Verification items for the finished model (mm, model axes). A direction names the side the tool comes from. Coordinates: 2 decimals unless noted, no trailing zeros. Order: outer loops, then holes, each group sorted by start corner. A loop starts at its lowest first (then second) coordinate and runs counter-clockwise, first axis right, second up. Notation, with made-up numbers: M 81.5,67 L 113.5,67 A14 cw 113.5,88 Z; hole C -12.75,14 d2. An arc over 180 degrees is marked long. Return JSON: item names as keys, results as strings. Group by question number.
1. Material ranges on line 1 along Y through (x, z) = (16, 1.55); line 2 along X through (y, z) = (-18, 3.2); line 3 along Y through (x, z) = (-15.5, 4.2), recorded low to high.
2. Gauge pin test, flat ends, axial feed: pin 1 (1.1 mm diameter, centred on x = 23, z = 2, fed in from -Y); pin 2 (3.5 mm diameter, centred on x = -16.02, y = 16.02, fed in from +Z); pin 3 (3 mm diameter, centred on y = -22.5, z = 2, fed in from +X). Record the tip position at first contact, or that the pin passes through.
3. Mould release check, pull along X, two halves, no side actions. Record for faces 1 (the cylindrical face through (-13.336, 16.616, 3.479)), 2 (the flat face through (-5.9, 11.4, 5)), 3 (the flat face through (-24.901, 0, 2)): +X half, -X half, draft (parallel to the pull), parting line (faces both ways), or undercut.
4. Section check C-C, the plane z = 1.15. Record the cut outline in (x, y), plus the area to 3 significant figures.
5. Section check B-B, the plane y = 0. Record the cut outline in (x, z).
6. Section check D-D, the plane x = 20. Record the cut outline in (y, z).
7. Section check A-A, the plane x = 7.5. Record the cut outline in (y, z), plus the area to 3 significant figures.
8. Set-up check for faces 4 (the cylindrical face through (-13.58, -17.29, 3.48)), 5 (the flat face through (24.901, 0, 2)), 6 (the flat face through (-17, -23, 3)), 7 (the flat face through (23, 17, 3)): record each of +Z, -Z, +X, -X, +Y, -Y from which the full face is reachable in a straight line by a thin tool's end or side.
Autodesk Inventor part; units mm, degrees
ref_plane "YZ Plane" through (0, 0, 0) normal (1, 0, 0) x (0, 1, 0)
ref_plane "XZ Plane" through (0, 0, 0) normal (0, 1, 0) x (-1, 0, 0)
ref_plane "XY Plane" through (0, 0, 0) normal (0, 0, 1) x (1, 0, 0)
sketch "Sketch1" plane through (0, 0, 0) normal (0, 0, 1) x (1, 0, 0)
  line L0 (-39.3843, 0) -> (62.0012, 0) construction
  line L1 (0, -36.6008) -> (0, 45.3001) construction
  line L2 (0, 0) -> (33.6, 33.6) construction
  line L3 (0, 0) -> (47.5176, 0) construction
  line L4 (0, 24.9006) -> (16.8, 24.9006)
  line L5 (16.8, 24.9006) -> (16.8, 21.2406)
  line L6 (16.8, 21.2406) -> (19.0203, 19.0203)
  line L7 (24.9006, 0) -> (24.9006, 16.8)
  line L8 (24.9006, 16.8) -> (21.2406, 16.8)
  line L9 (21.2406, 16.8) -> (19.0203, 19.0203)
  line L10 (0, 24.9006) -> (-16.8, 24.9006)
  line L11 (-16.8, 24.9006) -> (-16.8, 21.2406)
  line L12 (-16.8, 21.2406) -> (-19.0203, 19.0203)
  line L13 (-24.9006, 0) -> (-24.9006, 16.8)
  line L14 (-24.9006, 16.8) -> (-21.2406, 16.8)
  line L15 (-21.2406, 16.8) -> (-19.0203, 19.0203)
  line L16 (0, -24.9006) -> (16.8, -24.9006)
  line L17 (16.8, -24.9006) -> (16.8, -21.2406)
  line L18 (16.8, -21.2406) -> (19.0203, -19.0203)
  line L19 (24.9006, 0) -> (24.9006, -16.8)
  line L20 (24.9006, -16.8) -> (21.2406, -16.8)
  line L21 (21.2406, -16.8) -> (19.0203, -19.0203)
  line L22 (0, -24.9006) -> (-16.8, -24.9006)
  line L23 (-16.8, -24.9006) -> (-16.8, -21.2406)
  line L24 (-16.8, -21.2406) -> (-19.0203, -19.0203)
  line L25 (-24.9006, 0) -> (-24.9006, -16.8)
  line L26 (-24.9006, -16.8) -> (-21.2406, -16.8)
  line L27 (-21.2406, -16.8) -> (-19.0203, -19.0203)
  circle A0 centre (0, 0) radius 12.5
  dimension "d0" = 45
  dimension "d1" = 16.8
  dimension "d2" = 3.66
  dimension "d3" = 3.14
  dimension "d4" = 25
extrude "Extrusion1" add sketch "Sketch1" along normal blind 5
sketch "Sketch2" plane through (0, 0, 5) normal (0, 0, 1) x (1, 0, 0)
  circle A0 centre (0, 0) radius 12.5 construction
  line L0 (16.8, 24.9006) -> (-16.8, 24.9006) construction
  line L1 (-16.8, 24.9006) -> (-16.8, 21.2406) construction
  line L2 (-16.8, 21.2406) -> (-21.2406, 16.8) construction
  line L3 (-21.2406, 16.8) -> (-24.9006, 16.8) construction
  line L4 (-24.9006, 16.8) -> (-24.9006, -16.8) construction
  line L5 (-24.9006, -16.8) -> (-21.2406, -16.8) construction
  line L6 (-21.2406, -16.8) -> (-16.8, -21.2406) construction
  line L7 (-16.8, -21.2406) -> (-16.8, -24.9006) construction
  line L8 (-16.8, -24.9006) -> (16.8, -24.9006) construction
  line L9 (16.8, -24.9006) -> (16.8, -21.2406) construction
  line L10 (16.8, -21.2406) -> (21.2406, -16.8) construction
  line L11 (21.2406, -16.8) -> (24.9006, -16.8) construction
  line L12 (24.9006, -16.8) -> (24.9006, 16.8) construction
  line L13 (24.9006, 16.8) -> (21.2406, 16.8) construction
  line L14 (21.2406, 16.8) -> (16.8, 21.2406) construction
  line L15 (16.8, 21.2406) -> (16.8, 24.9006) construction
  circle A1 centre (16.0203, -16.0203) radius 2.1846 construction
  circle A2 centre (-16.0203, -16.0203) radius 2.1846 construction
  circle A3 centre (-16.0203, 16.0203) radius 2.1846 construction
  circle A4 centre (16.0203, 16.0203) radius 2.1846 construction
  circle A5 centre (0, 0) radius 14 construction
  line L16 (-19.0203, 17.0203) -> (-19.0203, -17.0203) construction
  arc A6 (-17.0203, 19.0203) -> (-19.0203, 17.0203) centre (-17.0203, 17.0203) ccw construction
  line L17 (17.0203, 19.0203) -> (-17.0203, 19.0203) construction
  arc A7 (19.0203, 17.0203) -> (17.0203, 19.0203) centre (17.0203, 17.0203) ccw construction
  line L18 (19.0203, -17.0203) -> (19.0203, 17.0203) construction
  arc A8 (17.0203, -19.0203) -> (19.0203, -17.0203) centre (17.0203, -17.0203) ccw construction
  line L19 (-17.0203, -19.0203) -> (17.0203, -19.0203) construction
  arc A9 (-19.0203, -17.0203) -> (-17.0203, -19.0203) centre (-17.0203, -17.0203) ccw construction
hole "Hole1" at (-16.0203, 16.0203, 5) at (16.0203, 16.0203, 5) at (16.0203, -16.0203, 5) at (-16.0203, -16.0203, 5) direction (0, 0, -1) diameter 2.8 end through all counterbore diameter 5.5 counterbore depth 3
sketch "Skizze3" plane through (0, 0, 5) normal (0, 0, 1) x (1, 0, 0)
  circle A0 centre (16.0203, -16.0203) radius 2.75 construction
  circle A1 centre (-16.0203, 16.0203) radius 2.75 construction
  circle A2 centre (16.0203, 16.0203) radius 2.75 construction
  circle A3 centre (-16.0203, -16.0203) radius 2.75 construction
  circle A4 centre (0, 0) radius 12.5 construction
  line L0 (16.8, 24.9006) -> (-16.8, 24.9006) construction
  line L1 (-16.8, 24.9006) -> (-16.8, 21.2406)
  line L2 (-16.8, 21.2406) -> (-21.2406, 16.8)
  line L3 (-21.2406, 16.8) -> (-24.9006, 16.8)
  line L4 (-24.9006, 16.8) -> (-24.9006, -16.8) construction
  line L5 (-24.9006, -16.8) -> (-21.2406, -16.8)
  line L6 (-21.2406, -16.8) -> (-16.8, -21.2406)
  line L7 (-16.8, -21.2406) -> (-16.8, -24.9006)
  line L8 (-16.8, -24.9006) -> (16.8, -24.9006) construction
  line L9 (16.8, -24.9006) -> (16.8, -21.2406)
  line L10 (16.8, -21.2406) -> (21.2406, -16.8)
  line L11 (21.2406, -16.8) -> (24.9006, -16.8)
  line L12 (24.9006, -16.8) -> (24.9006, 16.8) construction
  line L13 (24.9006, 16.8) -> (21.2406, 16.8)
  line L14 (21.2406, 16.8) -> (16.8, 21.2406)
  line L15 (16.8, 21.2406) -> (16.8, 24.9006)
  line L16 (-17, 25.1006) -> (17, 25.1006) construction
  line L17 (17, 25.1006) -> (17, 21.3235)
  line L18 (17, 21.3235) -> (21.3235, 17)
  line L19 (21.3235, 17) -> (25.1006, 17)
  line L20 (25.1006, 17) -> (25.1006, -17) construction
  line L21 (25.1006, -17) -> (21.3235, -17)
  line L22 (21.3235, -17) -> (17, -21.3235)
  line L23 (17, -21.3235) -> (17, -25.1006)
  line L24 (17, -25.1006) -> (-17, -25.1006) construction
  line L25 (-17, -25.1006) -> (-17, -21.3235)
  line L26 (-17, -21.3235) -> (-21.3235, -17)
  line L27 (-21.3235, -17) -> (-25.1006, -17)
  line L28 (-25.1006, -17) -> (-25.1006, 17) construction
  line L29 (-25.1006, 17) -> (-21.3235, 17)
  line L30 (-21.3235, 17) -> (-17, 21.3235)
  line L31 (-17, 21.3235) -> (-17, 25.1006)
  line L32 (-24.9006, 16.8) -> (-24.9006, 17)
  line L33 (-16.8, 24.9006) -> (-17, 24.9006)
  line L34 (16.8, 24.9006) -> (17, 24.9006)
  line L35 (24.9006, 16.8) -> (24.9006, 17)
  line L36 (24.9006, -16.8) -> (24.9006, -17)
  line L37 (16.8, -24.9006) -> (16.8, -21.2406)
  line L38 (16.8, -24.9006) -> (17, -24.9006)
  line L39 (-16.8, -24.9006) -> (-17, -24.9006)
  line L40 (-24.9006, -16.8) -> (-24.9006, -17)
  dimension "d14" = 0.2
extrude "IM_offset" add sketch "Skizze3" against normal up to surface (5 mm away)
properties part number "20_Cube_insert_Sample_holder_magnetic_v3"
Answers follow:
{
 "1": {"line 1": "-24.9 to -17.42, -14.62 to 14.62, 17.42 to 24.9", "line 2": "-20.32 to -17.93, -14.11 to 14.11, 17.93 to 20.32", "line 3": "-24.9 to -18.72, -13.32 to 13.32, 18.72 to 24.9"},
 "2": {"pin 1": "y = -17", "pin 2": "z = 2", "pin 3": "x = 17.32"},
 "3": {"face 1": "undercut", "face 2": "draft", "face 3": "-X half"},
 "4": {"outline": "M -24.9,-17 L -21.32,-17 L -17,-21.32 L -17,-24.9 L 17,-24.9 L 17,-21.32 L 21.32,-17 L 24.9,-17 L 24.9,17 L 21.32,17 L 17,21.32 L 17,24.9 L -17,24.9 L -17,21.32 L -21.32,17 L -24.9,17 Z; hole C -16.02,-16.02 d2.8; hole C -16.02,16.02 d2.8; hole C 0,0 d25; hole C 16.02,-16.02 d2.8; hole C 16.02,16.02 d2.8", "area": "1,750 mm^2"},
 "5": {"outline": "M -24.9,0 L -12.5,0 L -12.5,5 L -24.9,5 Z; M 12.5,0 L 24.9,0 L 24.9,5 L 12.5,5 Z"},
 "6": {"outline": "M -18.32,0 L 18.32,0 L 18.32,5 L -18.32,5 Z"},
 "7": {"outline": "M -24.9,0 L -10,0 L -10,5 L -24.9,5 Z; M 10,0 L 24.9,0 L 24.9,5 L 10,5 Z", "area": "149 mm^2"},
 "8": {"face 4": "+Z", "face 5": "+Z, -Z, +X, +Y, -Y", "face 6": "+Z, -Z, -X, -Y", "face 7": "+Z, -Z, +X, +Y"}
}
